```python
from build123d import *

# Parameters (mm, degrees)
SCHIZZO1_R                   = 30
ESTRUSIONE_ESTRUSIONE1_DEPTH = 8
SCHIZZO3_R                   = 4
TAGLIO_ESTRUSIONE1_DEPTH     = 9
RACCORDO1_R                  = 2


with BuildPart() as part:
    # Schizzo1 → Estrusione-Estrusione1 (new body)
    with BuildSketch(Plane(origin=(0, 0, 0), x_dir=(0, 0, -1), z_dir=(1, 0, 0))):
        Circle(SCHIZZO1_R)
    extrude(amount=ESTRUSIONE_ESTRUSIONE1_DEPTH)

    # Schizzo3 → Taglio-Estrusione1 (cut, through all)
    with BuildSketch(Plane(origin=(8, 0, 0), x_dir=(0, 0, -1), z_dir=(1, 0, 0))):
        Circle(SCHIZZO3_R)
    extrude(amount=-TAGLIO_ESTRUSIONE1_DEPTH, mode=Mode.SUBTRACT)

    # Raccordo1
    raccordo1_edges = [part.edges().sort_by_distance(p)[0] for p in [
        (0, 0, 30),
        (8, 0, 30),
    ]]
    fillet(raccordo1_edges, radius=RACCORDO1_R)


solid = part.part
```
CAD build for the part. Positions are in the model's coordinates, mm. Give positions to 0.01 mm unless a question says otherwise; leave off trailing zeros. Loops run counter-clockwise (first coordinate to the right, second up) from the corner with the lowest first, then second, coordinate; pieces in that order, holes last. Notation, with made-up numbers: M -30,-23.75 L 25,-23.75 A13 ccw 25,-1.75 Z; hole C 1,51.5 d2. An arc over 180 degrees is marked long. Use one line per item in the form item = value.
Item 1: Slice it at C-C (x = 3). List the corners of the cut face in (y, z), plus the area to 3 significant figures.
Determined:
outline = C 0,0 d60; hole C 0,0 d8
area = 2,780 mm2
Item 2: Two-plate mould, pull along Z, no slides. Class faces 1 (the face through (4.056, -3.905, 0.867)), 2 (the face through (0, -6, 0)), 3 (the face through (3.97, 1.32, 29.97)): pulls with the +Z half, pulls with the -Z half, needs draft (parallel to the pull), parting line crosses it, or undercut.
Determined:
face_1 = undercut
face_2 = needs draft
face_3 = parting line crosses it
Item 3: Slice it at A-A (y = 0). List the corners of the cut face in (x, z).
Determined:
outline = M 0,-28 A2 ccw 2,-30 L 6,-30 A2 ccw 8,-28 L 8,-4 L 0,-4 Z; M 0,4 L 8,4 L 8,28 A2 ccw 6,30 L 2,30 A2 ccw 0,28 Z
Item 4: Drill centre lines: probe 1 along Y at (x, z) = (6, 0); probe 2 along Y at (x, z) = (7.25, 1.5); probe 3 along Z at (x, y) = (4.25, 18.5). Where is each one in solid material? Low to high. Write a range as from..to.
Determined:
probe_1 = -30..-4, 4..30
probe_2 = -29.52..-3.71, 3.71..29.52
probe_3 = -23.62..23.62
Item 5: Flat gauge pins, fed straight in: pin 1 (1 mm diameter, centred on x = 4.5, z = -8, fed in from -Y); pin 2 (1 mm diameter, centred on x = 6.5, z = -18, fed in from -Y). Where does each tip first touch, or does it go through?
Determined:
pin_1 = -29.05
pin_2 = -24.31
